Input: part model. Units: mm. Frame: model coordinates. A direction names the side the tool comes from. Coordinates: 2 decimals unless noted, no trailing zeros. Write each loop counter-clockwise with the first axis right and the second up, starting at its lowest first coordinate (ties: lowest second). Pieces come first, ordered by that corner, then holes. Notation, with made-up numbers: (37, 74) - (54, 74) arc R28 cw to (54, 94) - close; hole circle Ø5 at (78, 15). An arc over 180 degrees is marked (long way). One line per question, with ' | ' between items. Start each with the question number.
1) Section query A-A on z = 16. Return loops of the section in (x, y).
2) Section query B-B on x = 2.8. Return loops of the section in (y, z), and give its area (3 significant figures).
3) Reachability of faces 1 (the cylindrical face through (3.538, -4.496, 18.56)), 2 (the flat face through (1, -5, 14)) from +Z, -Z, +X, -X, +Y, -Y: full face, straight path, thin tool, end or side. Return the list, or none.
4) Section query D-D on x = 1.35. Return loops of the section in (y, z), and give its area (3 significant figures).
5) Section query C-C on y = -1.75. Return loops of the section in (x, z), and give its area (3 significant figures).
6) Draft query along X for faces 3 (the flat face through (0, -2, 15)), 4 (the flat face through (0.2, -2.5, 12.574)), 5 (the cylindrical face through (1.69, -2.54, 13.81)). Return one class per face: released by +X, released by -X, zero draft, split by the parting line, or undercut.
7) Line query: line 1 (Z direction, x = 2.45, y = -2.4); line 2 (Y direction, x = 2.45, z = 17.75); line 3 (X direction, y = -4.65, z = 15.25). Output: solid intervals per line, ascending.
8) First-contact query: P1, Ø1.5, axis at x = 2.5, z = 15.5, coming from the -Y side. Flat tip, straight axial feed; report the tip coordinate or a pass-through.
```python
from build123d import *

# Parameters (mm, degrees)
F0_W     = 5
F0_H     = 5
F1_DEPTH = 5
F2_D     = 3
F3_R     = 2.25
F4_DEPTH = 2
F6_DEPTH = 1.5


with BuildPart() as f1:
    # F0 (on Front) → F1 (new body)
    with BuildSketch(Plane.XZ):
        with Locations((2.5, 15.0736845657)):
            Rectangle(F0_W, F0_H)
    extrude(amount=F1_DEPTH)

    # F2 (through all)
    with Locations(Plane(origin=(0, 0, 0), x_dir=(1, 0, 0), z_dir=(0, 1, 0))):
        with Locations((2.5, -15.0736845657)):
            Hole(F2_D / 2)

    # F3 (on face) → F4 (join)
    with BuildSketch(Plane.XY.offset(17.5736845657)):
        with Locations((2.5, -2.5)):
            Circle(F3_R)
    extrude(amount=F4_DEPTH)

    # F5 (on face) → F6 (join)
    with BuildSketch(Plane(origin=(0, 0, 12.5736845657), x_dir=(1, 0, 0), z_dir=(0, 0, -1))):
        with BuildLine():
            Line((2.5, 2.5), (2.5, 4.5))
            ThreePointArc((2.5, 4.5), (1.0857864376, 3.9142135624), (0.5, 2.5))
            Line((0.5, 2.5), (2.5, 2.5))
        make_face()
        with BuildLine():
            ThreePointArc((4.5, 2.5), (3.9142135624, 3.9142135624), (2.5, 4.5))
            Line((2.5, 4.5), (2.5, 2.5))
            Line((2.5, 2.5), (4.5, 2.5))
        make_face()
        with BuildLine():
            Line((4.5, 2.5), (2.5, 2.5))
            Line((2.5, 2.5), (2.5, 0.5))
            ThreePointArc((2.5, 0.5), (3.9142135624, 1.0857864376), (4.5, 2.5))
        make_face()
        with BuildLine():
            Line((2.5, 0.5), (2.5, 2.5))
            Line((2.5, 2.5), (0.5, 2.5))
            ThreePointArc((0.5, 2.5), (1.0857864376, 1.0857864376), (2.5, 0.5))
        make_face()
    extrude(amount=F6_DEPTH)


solid = f1.part
```
Answer key:
1) outline: (0, -5) - (1.32, -5) - (1.32, 0) - (0, 0) - close; (3.68, -5) - (5, -5) - (5, 0) - (3.68, 0) - close
2) outline: (-5, 12.57) - (-4.48, 12.57) - (-4.48, 11.07) - (-0.52, 11.07) - (-0.52, 12.57) - (0, 12.57) - (0, 13.6) - (-5, 13.6) - close; (-5, 16.54) - (0, 16.54) - (0, 17.57) - (-0.27, 17.57) - (-0.27, 19.57) - (-4.73, 19.57) - (-4.73, 17.57) - (-5, 17.57) - close | area: 25.2 mm²
3) face 1: +Z | face 2: +Z, -Z, +X, -X, -Y
4) outline: (-5, 12.57) - (-4.14, 12.57) - (-4.14, 11.07) - (-0.86, 11.07) - (-0.86, 12.57) - (0, 12.57) - (0, 14.11) - (-5, 14.11) - close; (-5, 16.04) - (0, 16.04) - (0, 17.57) - (-0.57, 17.57) - (-0.57, 19.57) - (-4.43, 19.57) - (-4.43, 17.57) - (-5, 17.57) - close | area: 28.0 mm²
5) outline: (0, 12.57) - (0.65, 12.57) - (0.65, 11.07) - (4.35, 11.07) - (4.35, 12.57) - (5, 12.57) - (5, 17.57) - (4.62, 17.57) - (4.62, 19.57) - (0.38, 19.57) - (0.38, 17.57) - (0, 17.57) - close; hole circle Ø3 at (2.5, 15.07) | area: 32.0 mm²
6) face 3: released by -X | face 4: zero draft | face 5: undercut
7) line 1: 11.07 to 13.57, 16.57 to 19.57 | line 2: -4.75 to -0.25 | line 3: 0 to 1.01, 3.99 to 5
8) P1: through
